Check sheet for the modelled part. Datum: model origin and axes. Units: mm. A direction names the side the tool comes from. Round coordinates to 2 decimals unless told otherwise and drop trailing zeros. Write each loop counter-clockwise with the first axis right and the second up, starting at its lowest first coordinate (ties: lowest second). Pieces come first, ordered by that corner, then holes. Notation, with made-up numbers: M -6,-13 L 45,-13 A27 ccw 45,26 Z; hole C 66.25,77 d5. An arc over 180 degrees is marked long. One line per item, written item: value.
from build123d import *

# Parameters (mm, degrees)
F0_R        = 2
F1_DEPTH    = 3
F3_DEPTH    = 21.5
F4_SIZE     = 2.99999
F5_R        = 1
F6_T4_DEPTH = 60.8867319519
F6_T9_DEPTH = 60.8867319519


# Not quite as in the source:
# - a fillet or chamfer that OpenCascade refuses, or shapes differently, is made with other operations: its cross-section is extruded or revolved along the edge and cut away or added
# - a fillet or chamfer is up to 0.001 mm smaller than in the source, because OpenCascade refuses the exact size


with BuildPart() as f1:
    # F0 (on Top) → F1 (new body)
    with BuildSketch(Plane.XY):
        Polygon((0, -80), (0, 0), (-80, 0), (-80, -25.4), (-25.4, -80), align=None)
        with Locations((-12.7, -65)):
            Circle(F0_R, mode=Mode.SUBTRACT)
        with Locations((-70, -12.7)):
            Circle(F0_R, mode=Mode.SUBTRACT)
        with Locations((-12.7, -35)):
            Circle(F0_R, mode=Mode.SUBTRACT)
        with Locations((-40, -12.7)):
            Circle(F0_R, mode=Mode.SUBTRACT)
    extrude(amount=F1_DEPTH)

    # F2 (on face) → F3 (join)
    with BuildSketch(Plane.XY.offset(3)):
        Polygon((-25.4, -25.4), (-80, -25.4), (-78, -27.4), (-27.4, -27.4), (-27.4, -78), (-25.4, -80), align=None)
    extrude(amount=F3_DEPTH)

    # F4 (size 3 in the source; OpenCascade refuses exactly that, so slightly less here)
    f4_edges = [f1.edges().sort_by_distance(p)[0] for p in [
        (-40, 0, 0),
        (0, -40, 0),
    ]]
    chamfer(f4_edges, length=F4_SIZE)

    # F5
    f5_edges = [f1.edges().sort_by_distance(p)[0] for p in [
        (-25.4, -25.4, 13.75),
    ]]
    fillet(f5_edges, radius=F5_R)

    # F6: chamfer of 2 on 2 edges, made by hand


with BuildPart() as f6_tool2:
    # F6_s3 → F6_t4 (new body)
    with BuildSketch(Plane.YZ.offset(-83.1433659759)):
        Polygon((-25.4, 24.5), (-27.4, 22.5), (-27.4, 24.5), align=None)
    extrude(amount=F6_T4_DEPTH)

    split(bisect_by=Plane(origin=(-24.95, 0, 24.95), x_dir=(0, 1, 0), z_dir=(-0.7071067812, 0, 0.7071067812)), keep=Keep.TOP)


with BuildPart() as f1_1:
    add(f1.part)

    # F6_t1: cut F6_tool2
    add(f6_tool2.part, mode=Mode.SUBTRACT)


with BuildPart() as f6_tool7:
    # F6_s8 → F6_t9 (new body)
    with BuildSketch(Plane.XZ.offset(22.2566340241)):
        Polygon((-25.4, 24.5), (-27.4, 22.5), (-27.4, 24.5), align=None)
    extrude(amount=F6_T9_DEPTH)

    split(bisect_by=Plane(origin=(0, -24.95, 24.95), x_dir=(1, 0, 0), z_dir=(0, -0.7071067812, 0.7071067812)), keep=Keep.TOP)


with BuildPart() as f1_2:
    add(f1_1.part)

    # F6_t6: cut F6_tool7
    add(f6_tool7.part, mode=Mode.SUBTRACT)


solid = f1_2.part
Q1. Access from +Z, -Z, +X, -X, +Y, -Y to the whole of each face (thin tool, end or side, straight path). Record for faces 1 (the flat face through (-32, -22, 3)), 2 (the flat face through (-25.4, -54, 14)), 3 (the flat face through (-53, -25.4, 14)), 4 (the flat face through (-53.2, -26.4, 23.5)).
Completed:
face 1: +Z, +X, +Y
face 2: +Z, +X, +Y, -Y
face 3: +Z, +X, -X, +Y
face 4: +Z, -X, -Y
Q2. Sectioned sample at B-B on x = -12.7. State how many separate pieces and enclosed holes the cut face has, and give its area (4 significant figures).
Completed:
separate pieces: 3
enclosed holes: 0
area: 211.5 mm^2
Q3. Scan lines: line 1 (Y direction, x = -12.7, z = 2.1); line 2 (Y direction, x = -12.7, z = 2.2); line 3 (Z direction, x = -48.5, y = -43). Record each from-to range of solid material in increasing order. Write a range as [from, to].
Completed:
line 1: [-80, -67], [-63, -37], [-33, -0.9]
line 2: [-80, -67], [-63, -37], [-33, -0.8]
line 3: [0, 3]
Q4. Depth check by flat-ended pin: P1, Ø1, axis at x = -18.5, y = -67.5, coming from the -Z side; P2, Ø5, axis at x = -40, y = -12.7, coming from the +Z side; P3, Ø6, axis at x = -45.5, z = 12, coming from the -Y side; P4, Ø12, axis at x = -65, z = 9.5, coming from the +Y side. Enter the tip coordinate at first touch or a pass-through.
Completed:
P1: z = 0
P2: z = 3
P3: y = -27.4
P4: y = -25.4
Q5. Draft check along Y on faces 5 (the cylindrical face through (-11.777, -36.774, 1.479)), 6 (the flat face through (-27.4, -52, 13)), 7 (the cylindrical face through (-41.6, -13.9, 1.5)), 8 (the flat face through (-52.8, -52.6, 2.2)). Enter one of: pulls with the +Y half, pulls with the -Y half, needs draft (parallel to the pull), parting line crosses it, or undercut.
Completed:
face 5: undercut
face 6: needs draft
face 7: undercut
face 8: pulls with the -Y half
Q6. Sectioned sample at D-D on z = 11.75. Enter the section's corners in (x, y), and give its area (3 significant figures).
Completed:
outline: M -80,-25.4 L -78,-27.4 L -27.4,-27.4 L -27.4,-78 L -25.4,-80 L -25.4,-26.4 A1 ccw -26.4,-25.4 Z
area: 210 mm^2
